The model under review builds one solid part; all positions refer to its coordinate system, in mm. A direction names the side the tool comes from. Round coordinates to 2 decimals unless told otherwise and drop trailing zeros. Order: outer loops, then holes, each group sorted by start corner. A loop starts at its lowest first (then second) coordinate and runs counter-clockwise, first axis right, second up. Notation, with made-up numbers: M 21.5,37.5 L 50.5,37.5 A21 cw 50.5,65.5 Z; hole C 61.25,26 d11. An arc over 180 degrees is marked long. Answer as a JSON object with one key per item and string values. Group by question number.
1) Consider section D-D, the plane y = -212.5. Write out the cut boundary in (x, z), then the cut area to 3 significant figures.
2) Consider section A-A, the plane z = -118. Write out the cut boundary in (x, y).
3) Insertion check: pin 1 Ø24 at (x, z) = (188, 55.5) entering from -Y. The pin has a flat end and moves straight along its axis. Give the tip position at first contact, or say it passes through.
4) For faces 1 (the flat face through (-3, -355.385, -108)), 2 (the flat face through (-263, 75, 40)), 3 (the flat face through (130, 96, 40)), 4 (the flat face through (-310, 0, 39)), list the 3-axis set-ups (+Z, -Z, +X, -X, +Y, -Y) from which the entire face can be reached by the end or side of a thin tool; tool diameter is ignored.
5) Consider section C-C, the plane x = 342. Write out the cut boundary in (y, z).
6) The part is to be moulded in two halves that separate along Y. For faces 5 (the flat face through (125, 91, 39)), 6 (the flat face through (-5, 187, 75)), 7 (the flat face through (-277, 80, 39)), say which applies: +Y half, -Y half, draft (parallel to the pull), parting line (faces both ways), or undercut.
7) To check wall thickness, follow line 1 (X direction, y = -201.5, z = -75); line 2 (X direction, y = 118, z = 9); line 3 (Z direction, x = 199.5, y = 181). State the ranges of each line that lie inside material, in increasing order.
8) Consider section B-B, the plane x = -101.5. Write out the cut boundary in (y, z), then the cut area to 3 significant figures.
```python
from build123d import *

# Parameters (mm, degrees)
EXTRUDE_1_DEPTH     = 80
SKETCH_2_W          = 80
SKETCH_2_H          = 80
SKETCH_2_W_2        = 70
SKETCH_2_H_2        = 70
EXTRUDE_2_DEPTH     = 385
SKETCH_4_W          = 900
SKETCH_4_H          = 80
EXTRUDE_3_DEPTH     = 80
EXTRUDE_5_DEPTH     = 40
SKETCH_8_W          = 70
SKETCH_8_H          = 70
CUT_EXTRUDE_1_DEPTH = 901


with BuildPart() as part:
    # Sketch 1 → Extrude 1 (new body)
    with BuildSketch(Plane.XY):
        Polygon((-125, 180), (125, 180), (125, 0), (325, 0), (325, 80), (205, 80), (205, 260), (-205, 260), (-205, 80), (-325, 80), (-325, 0), (-125, 0), align=None)
    extrude(amount=EXTRUDE_1_DEPTH)

    # Sketch 2 → Extrude 2 (add, along a direction that is not the sketch's normal)
    with BuildSketch(Plane.XZ):
        with Locations((-255, 40)):
            Rectangle(SKETCH_2_W, SKETCH_2_H)
        with Locations((-255, 40)):
            Rectangle(SKETCH_2_W_2, SKETCH_2_H_2, mode=Mode.SUBTRACT)
        with Locations((255, 40)):
            Rectangle(SKETCH_2_W, SKETCH_2_H)
        with Locations((255, 40)):
            Rectangle(SKETCH_2_W_2, SKETCH_2_H_2, mode=Mode.SUBTRACT)
    extrude(amount=EXTRUDE_2_DEPTH, dir=(0, -0.923076923, -0.384615385))

    # Sketch 4 → Extrude 3 (add)
    with BuildSketch(Plane.XZ.offset(355.384615385)):
        with Locations((125, -108.076923077)):
            Rectangle(SKETCH_4_W, SKETCH_4_H)
    extrude(amount=EXTRUDE_3_DEPTH)

    # Sketch 6 → Extrude 5 (add)
    with BuildSketch(Plane.XY.offset(20)):
        Polygon((-205, 130), (-255, 80), (-205, 80), align=None)
        Polygon((205, 130), (255, 80), (205, 80), align=None)
    extrude(amount=EXTRUDE_5_DEPTH)

    # Sketch 8 → Cut-Extrude 1 (cut, through all)
    with BuildSketch(Plane.ZY.offset(325)):
        with Locations((-108.076923077, -395.384615385)):
            Rectangle(SKETCH_8_W, SKETCH_8_H)
    extrude(amount=-CUT_EXTRUDE_1_DEPTH, mode=Mode.SUBTRACT)

    # Sweep 1: sweep along a path in Sketch 10
    with BuildLine(Plane(origin=(0, 0, 40), x_dir=(-1, 0, 0), z_dir=(0, 0, -1))) as sweep_1_path:
        Line((-325, 40), (-165, 40))
        Line((-165, 40), (-165, 220))
        Line((-165, 220), (165, 220))
        Line((165, 220), (165, 40))
        Line((165, 40), (325, 40))
    # Sketch 9 → Sweep 1 (sweep, cut)
    with BuildSketch(Plane(origin=(325, 0, 0), x_dir=(0, 0, -1), z_dir=(1, 0, 0))):
        Polygon((-5, 5), (-5, 75), (-20, 75), (-60, 75), (-75, 75), (-75, 5), align=None)
    sweep(path=sweep_1_path.line, transition=Transition.RIGHT, mode=Mode.SUBTRACT)


solid = part.part
```
Results list:
{
 "1": {"outline": "M -295,-88.54 L -215,-88.54 L -215,-8.54 L -295,-8.54 Z; M 215,-88.54 L 295,-88.54 L 295,-8.54 L 215,-8.54 Z; hole M -290,-83.54 L -220,-83.54 L -220,-13.54 L -290,-13.54 Z; hole M 220,-83.54 L 290,-83.54 L 290,-13.54 L 220,-13.54 Z", "area": "3,000 mm^2"},
 "2": {"outline": "M -325,-435.38 L 575,-435.38 L 575,-430.38 L -325,-430.38 Z; M -325,-360.38 L 575,-360.38 L 575,-355.38 L 295,-355.38 L 295,-283.2 L 215,-283.2 L 215,-355.38 L -215,-355.38 L -215,-283.2 L -295,-283.2 L -295,-355.38 L -325,-355.38 Z; hole M -290,-355.38 L -220,-355.38 L -220,-295.2 L -290,-295.2 Z; hole M 220,-355.38 L 290,-355.38 L 290,-295.2 L 220,-295.2 Z"},
 "3": {"pin 1": "y = 0"},
 "4": {"face 1": "+Z, -Z, +Y", "face 2": "-X", "face 3": "none", "face 4": "+Z, -Z, -X, -Y"},
 "5": {"outline": "M -435.38,-148.08 L -355.38,-148.08 L -355.38,-68.08 L -435.38,-68.08 Z; hole M -430.38,-143.08 L -360.38,-143.08 L -360.38,-73.08 L -430.38,-73.08 Z"},
 "6": {"face 5": "draft", "face 6": "undercut", "face 7": "+Y half"},
 "7": {"line 1": "-295 to -290, -220 to -215, 215 to 220, 290 to 295", "line 2": "-205 to -200, -130 to -125, 125 to 130, 200 to 205", "line 3": "0 to 5, 75 to 80"},
 "8": {"outline": "M -435.38,-148.08 L -355.38,-148.08 L -355.38,-68.08 L -435.38,-68.08 Z; M 180,0 L 260,0 L 260,80 L 180,80 Z; hole M -430.38,-143.08 L -360.38,-143.08 L -360.38,-73.08 L -430.38,-73.08 Z; hole M 185,5 L 255,5 L 255,75 L 185,75 Z", "area": "3,000 mm^2"}
}
